```python
from build123d import *

# Parameters (mm, degrees)
SKETCH_1_R          = 65.5
EXTRUDE_1_DEPTH     = 3
SKETCH_2_R          = 2.45
EXTRUDE_2_DEPTH     = 4
SKETCH_3_R          = 10.65
CUT_EXTRUDE_1_DEPTH = 93.717312299


with BuildPart() as part:
    # 草图1 → 凸台-拉伸1 (new body)
    with BuildSketch(Plane.XY):
        Circle(SKETCH_1_R)
    extrude(amount=-EXTRUDE_1_DEPTH)

    # 草图2 → 凸台-拉伸2 (add)
    with BuildSketch(Plane.XY):
        with Locations((-63, 0)):
            Circle(SKETCH_2_R)
        with Locations((-31.5, 54.559600438)):
            Circle(SKETCH_2_R)
        with Locations((31.5, 54.559600438)):
            Circle(SKETCH_2_R)
        with Locations((63, 0)):
            Circle(SKETCH_2_R)
        with Locations((31.5, -54.559600438)):
            Circle(SKETCH_2_R)
        with Locations((-31.5, -54.559600438)):
            Circle(SKETCH_2_R)
    extrude(amount=EXTRUDE_2_DEPTH)

    # 草图3 → 切除-拉伸1 (cut, through all)
    with BuildSketch(Plane.XY):
        Circle(SKETCH_3_R)
    extrude(amount=-CUT_EXTRUDE_1_DEPTH, mode=Mode.SUBTRACT)


solid = part.part
```
Input: part model. Units: mm. Frame: model coordinates. A direction names the side the tool comes from. Give positions to 0.01 mm unless a question says otherwise; leave off trailing zeros. Loops run counter-clockwise (first coordinate to the right, second up) from the corner with the lowest first, then second, coordinate; pieces in that order, holes last.
1) Mould query, pull axis X, two halves, no side actions, for faces 1 (the cylindrical face through (62.475, 19.674, -1.479)), 2 (the cylindrical face through (10.158, 3.199, -1.479)), 3 (the flat face through (31, -55, 4)), 4 (the cylindrical face through (-30.183, 56.625, 1.972)). Classes: released by +X, released by -X, zero draft, split by the parting line, or undercut.
A:
face 1: split by the parting line
face 2: undercut
face 3: zero draft
face 4: undercut
2) Section query D-D on z = -1.75. Return the cut outline in (x, y), and give its area (3 significant figures).
A:
outline: circle Ø131 at (0, 0); hole circle Ø21.3 at (0, 0)
area: 13,100 mm2
3) Line query: L1, parallel to Y at x = 0, z = -0.7; L2, parallel to Z at x = 9.5, y = 29.5; L3, parallel to Y at x = 5.5, z = -0.75. Output: solid intervals per line, ascending.
A:
L1: y = -65.5 to -10.65, 10.65 to 65.5
L2: z = -3 to 0
L3: y = -65.27 to -9.12, 9.12 to 65.27
4) Section query A-A on y = 0. Return the cut outline in (x, z).
A:
outline: (-65.5, -3) - (-10.65, -3) - (-10.65, 0) - (-60.55, 0) - (-60.55, 4) - (-65.45, 4) - (-65.45, 0) - (-65.5, 0) - close; (10.65, -3) - (65.5, -3) - (65.5, 0) - (65.45, 0) - (65.45, 4) - (60.55, 4) - (60.55, 0) - (10.65, 0) - close
5) Reachability of faces 5 (the flat face through (31, 55, 4)), 6 (the cylindrical face through (-60.663, 0.736, 1.972)) from +Z, -Z, +X, -X, +Y, -Y: full face, straight path, thin tool, end or side. Return the list, or none.
A:
face 5: +Z, +X, -X, +Y, -Y
face 6: +Z
6) Section query B-B on x = 0. Return the cut outline in (y, z).
A:
outline: (-65.5, -3) - (-10.65, -3) - (-10.65, 0) - (-65.5, 0) - close; (10.65, -3) - (65.5, -3) - (65.5, 0) - (10.65, 0) - close
7) Section query C-C on x = -63. Return the cut outline in (y, z), and give its area (3 significant figures).
A:
outline: (-17.92, -3) - (17.92, -3) - (17.92, 0) - (2.45, 0) - (2.45, 4) - (-2.45, 4) - (-2.45, 0) - (-17.92, 0) - close
area: 127 mm2
8) Contact query for flat-ended pins moving along their axis: pin 1 (2 mm diameter, centred on y = -22, z = 0, fed in from +X); pin 2 (1.5 mm diameter, centred on y = -18, z = -0.5, fed in from -X); pin 3 (1 mm diameter, centred on x = 4.5, z = -0.5, fed in from -Y). Output: stop coordinate, or through.
A:
pin 1: stops at x = 62.04
pin 2: stops at x = -63.19
pin 3: stops at y = -65.38
